For this review, take the finished solid that the model builds, in its own axes (mm). A direction names the side the tool comes from. Coordinates: 2 decimals unless noted, no trailing zeros. Loops run counter-clockwise (first coordinate to the right, second up) from the corner with the lowest first, then second, coordinate; pieces in that order, holes last. Notation, with made-up numbers: (-9.75, 22) - (47.25, 22) arc R22 cw to (47.25, 35) - close; hole circle Ø6 at (12, 29.5). An arc over 180 degrees is marked (long way). Answer as a JSON object with one key per item and string values. Group by question number.
Item 1: Mouldability with a two-part tool opening along Y and no side actions: class faces 1 (the flat face through (2, -77.788, -19)), 2 (the flat face through (2, 67, -30.162)), 3 (the flat face through (2, 79, 4.762)) as released by +Y, released by -Y, zero draft, split by the parting line, or undercut.
Item 2: We need section B-B (y = 46.5). Give the boundary of the cut face in (x, z) (1 decimal), then the cut area to 3 significant figures.
Item 3: Clearance check with flat-ended pins moving along their axes: pin 1 (1 mm diameter, centred on x = 1, y = -45.5, fed in from -Z); pin 2 (1.5 mm diameter, centred on x = 1, z = 21.5, fed in from -Y); pin 3 (2 mm diameter, centred on y = 15, z = -21.5, fed in from -X). State where each tip first meets the part, or that it passes through.
Item 4: Tool access review of faces 4 (the flat face through (2, -3, -33.338)), 5 (the flat face through (2, 79, -4.762)), 6 (the flat face through (2, -77.788, 19)), 7 (the flat face through (2, -1, 33.338)), 8 (the flat face through (2, -1.588, -17)): name each direction out of +Z, -Z, +X, -X, +Y, -Y from which nothing blocks a thin tool from reaching the whole face with its end or side.
Item 5: We need section A-A (z = -1.5). Give the boundary of the cut face in (x, y) (1 decimal), then the cut area to 3 significant figures.
Item 6: To check wall thickness, follow line 1 (Y direction, x = 1.8, z = -12); line 2 (Y direction, x = 2.4, z = -19); line 3 (Z direction, x = 0.5, y = 11.5). State the ranges of each line that lie inside material, in increasing order.
from build123d import *

# Parameters (mm, degrees)
F0_W     = 161.925
F0_H     = 66.675
F1_DEPTH = 3.175
F2_W     = 3.175
F2_H     = 9.525
F3_DEPTH = 3.176
F4_W     = 9.525
F4_H     = 3.175
F5_DEPTH = 3.176
F6_W     = 3.175
F6_H     = 33.3375
F7_DEPTH = 3.176


with BuildPart() as f1:
    # F0 (on Right) → F1 (new body)
    with BuildSketch(Plane.YZ):
        Rectangle(F0_W, F0_H)
    extrude(amount=F1_DEPTH)

    # F2 (on face) → F3 (cut, through all)
    with BuildSketch(Plane.YZ.offset(3.175)):
        with Locations((-79.375, -19.05)):
            Rectangle(F2_W, F2_H)
        with Locations((-79.375, 0)):
            Rectangle(F2_W, F2_H)
        with Locations((-79.375, 19.05)):
            Rectangle(F2_W, F2_H)
        with Locations((79.375, -19.05)):
            Rectangle(F2_W, F2_H)
        with Locations((79.375, 0)):
            Rectangle(F2_W, F2_H)
        with Locations((79.375, 19.05)):
            Rectangle(F2_W, F2_H)
    extrude(amount=-F3_DEPTH, mode=Mode.SUBTRACT)

    # F4 (on face) → F5 (cut, through all)
    with BuildSketch(Plane.YZ.offset(3.175)):
        with Locations((-66.675, -31.75)):
            Rectangle(F4_W, F4_H)
        with Locations((-47.625, -31.75)):
            Rectangle(F4_W, F4_H)
        with Locations((-28.575, -31.75)):
            Rectangle(F4_W, F4_H)
        with Locations((-9.525, -31.75)):
            Rectangle(F4_W, F4_H)
        with Locations((9.525, -31.75)):
            Rectangle(F4_W, F4_H)
        with Locations((28.575, -31.75)):
            Rectangle(F4_W, F4_H)
        with Locations((47.625, -31.75)):
            Rectangle(F4_W, F4_H)
        with Locations((66.675, -31.75)):
            Rectangle(F4_W, F4_H)
    extrude(amount=-F5_DEPTH, mode=Mode.SUBTRACT)

    # F6 (on face) → F7 (cut, through all)
    with BuildSketch(Plane.YZ.offset(3.175)):
        with Locations((0, -16.66875)):
            Rectangle(F6_W, F6_H)
    extrude(amount=-F7_DEPTH, mode=Mode.SUBTRACT)


solid = f1.part
Check sheet entries:
{
 "1": {"face 1": "released by -Y", "face 2": "undercut", "face 3": "zero draft"},
 "2": {"outline": "(0, -30.2) - (3.2, -30.2) - (3.2, 33.3) - (0, 33.3) - close", "area": "202 mm2"},
 "3": {"pin 1": "stops at z = -30.16", "pin 2": "stops at y = -77.79", "pin 3": "stops at x = 0"},
 "4": {"face 4": "-Z, +X, -X, +Y, -Y", "face 5": "+X, -X, +Y", "face 6": "+X, -X, -Y", "face 7": "+Z, +X, -X, +Y, -Y", "face 8": "-Z, +X, -X"},
 "5": {"outline": "(0, -77.8) - (3.2, -77.8) - (3.2, -1.6) - (0, -1.6) - close; (0, 1.6) - (3.2, 1.6) - (3.2, 77.8) - (0, 77.8) - close", "area": "484 mm2"},
 "6": {"line 1": "y = -80.96 to -1.59, 1.59 to 80.96", "line 2": "y = -77.79 to -1.59, 1.59 to 77.79", "line 3": "z = -30.16 to 33.34"}
}
